Check sheet for the drawn part. Datum: minimum x, y, z corner. Units: mm. Coordinates: 2 decimals unless noted, no trailing zeros. Write each loop counter-clockwise with the first axis right and the second up, starting at its lowest first coordinate (ties: lowest second). Pieces come first, ordered by that corner, then holes. Notation, with made-up numbers: (-15.75, 71.25) -> (0.25, 71.25) arc R26 cw to (0.25, 109.25) -> close; hole circle Ø6 at (-27.75, 49). An arc over 180 degrees is marked (long way). Write each question's results on one line, items separated by ' | '. Start each with the question number.
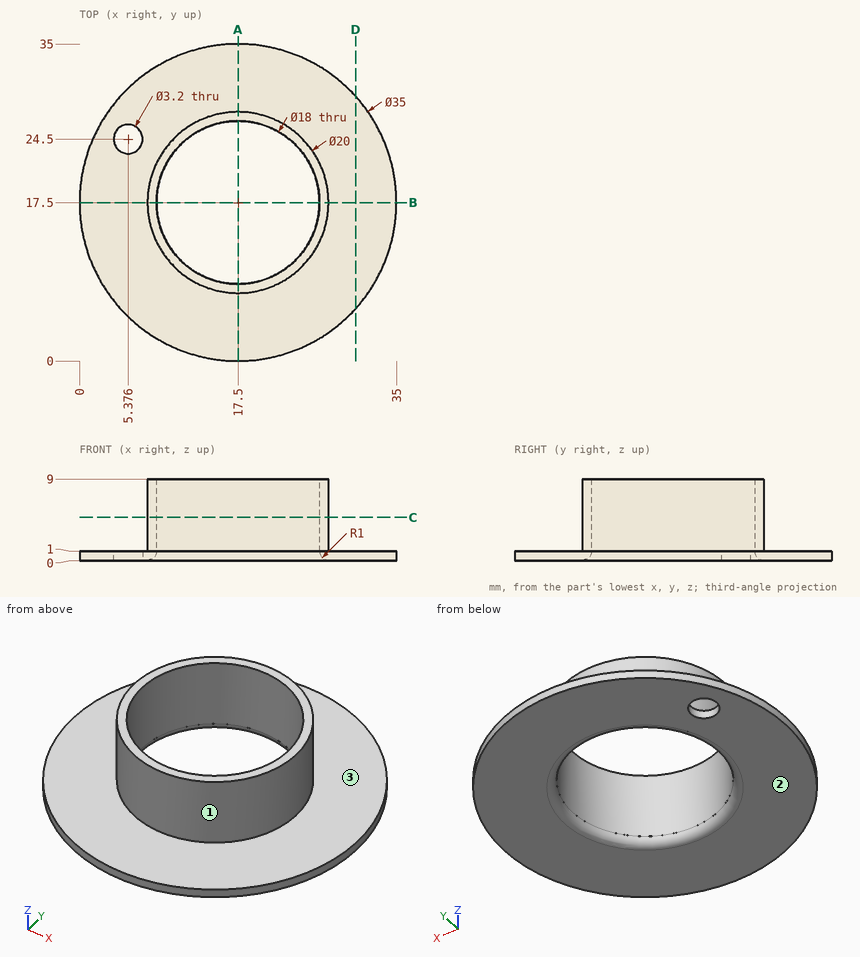
1. Mould release check, pull along Z, two halves, no side actions. Record for the marked faces 1, 2 and 3: +Z half, -Z half, draft (parallel to the pull), parting line (faces both ways), or undercut.
2. Sectioned sample at A-A on x = 17.5. Record the cut outline in (y, z).
3. Sectioned sample at C-C on z = 4.75. Record the cut outline in (x, y).
4. Sectioned sample at D-D on x = 30.5. Record the cut outline in (y, z) (1 decimal).
5. Material ranges on probe 1 along Y at (x, z) = (17.5, 1.05); probe 2 along Z at (x, y) = (7, 6.5); probe 3 along Y at (x, z) = (13.5, 7) (1 decimal), recorded low to high. Write a range as from..to.
6. Depth check by flat-ended pin: pin 1 Ø1.5 at (y, z) = (21, 3) entering from -X (1 decimal); pin 2 Ø1.9 at (x, y) = (5.38, 24.5) entering from +Z (1 decimal); pin 3 Ø1 at (x, z) = (19.5, 5) entering from -Y; pin 4 Ø6 at (x, y) = (10, 20.5) entering from -Z. Enter the tip coordinate at first touch or a pass-through.
Computed values:
1) face 1: draft | face 2: -Z half | face 3: +Z half
2) outline: (0, 0) -> (7.5, 0) arc R1 ccw to (8.5, 1) -> (8.5, 9) -> (7.5, 9) -> (7.5, 1) -> (0, 1) -> close; (26.5, 1) arc R1 ccw to (27.5, 0) -> (35, 0) -> (35, 1) -> (27.5, 1) -> (27.5, 9) -> (26.5, 9) -> close
3) outline: circle Ø20 at (17.5, 17.5); hole circle Ø18 at (17.5, 17.5)
4) outline: (5.8, 0) -> (29.2, 0) -> (29.2, 1) -> (5.8, 1) -> close
5) probe 1: y = 7.5..8.5, 26.5..27.5 | probe 2: z = 0..1 | probe 3: y = 8.3..9.4, 25.6..26.7
6) pin 1: stops at x = 7.9 | pin 2: passes through | pin 3: stops at y = 7.61 | pin 4: stops at z = 0
